Autodesk Fusion 360 part; units mm, degrees
sketch "Sketch1" plane through (0, 0, 0) normal (0, 1, 0) x (1, 0, 0)
  line L0 (-40.005, 0) -> (40.005, 0)
  line L1 (0, -29.21) -> (0, 0) construction
  line L2 (-1.524, -55.2004) -> (-1.524, -58.3802)
  line L3 (1.524, -55.2004) -> (1.524, -58.3802)
  line L4 (-1.524, -56.7903) -> (1.524, -56.7903) construction
  arc A0 (1.524, -55.2004) -> (-1.524, -55.2004) centre (0, -29.21) ccw
  arc A1 (40.005, 0) -> (29.1884, -28.0872) centre (67.2603, -26.6226) ccw
  arc A2 (-29.1884, -28.0872) -> (-40.005, 0) centre (-67.2603, -26.6226) ccw
  arc A3 (1.524, -58.3802) -> (29.1884, -28.0872) centre (0, -29.21) ccw
  arc A4 (-29.1884, -28.0872) -> (-1.524, -58.3802) centre (0, -29.21) ccw
  dimension "d1" = 52.07
  dimension "d2" = 29.21
  dimension "d3" = 80.01
  dimension "d4" = 58.42
  dimension "d5" = 3.048
  dimension "d7" = 38.1
extrude "Extrude1" add sketch "Sketch1" along normal blind 25.4
sketch "Sketch2" plane through (0, 0, 0) normal (0, 0, 1) x (1, 0, 0)
  circle A0 centre (0, 12.7) radius 3.302
  line L0 (-1.524, 25.4) -> (-29.21, 25.4)
  line L1 (-1.524, 0) -> (-29.21, 0)
  line L2 (-5.6643, 25.4) -> (-5.6643, 0) construction
  line L3 (-5.6643, 12.7) -> (0, 12.7) construction
  line L4 (1.524, 0) -> (1.524, 25.4) construction
  line L5 (-1.524, 0) -> (-1.524, 25.4) construction
  line L6 (0, 12.7) -> (0, 14.224) construction
  line L7 (0, 14.224) -> (-1.524, 14.224) construction
  line L8 (0, 14.224) -> (1.524, 14.224) construction
  dimension "d10" = 6.604
extrude "Extrude2" cut sketch "Sketch2" along normal blind 65.6387 and the other way blind -9.7561
Work out the finished part from the listing and answer in its coordinate system (mm). A direction names the side the tool comes from. Coordinates: 2 decimals unless noted, no trailing zeros. Write each loop counter-clockwise with the first axis right and the second up, starting at its lowest first coordinate (ties: lowest second). Pieces come first, ordered by that corner, then holes. Notation, with made-up numbers: (-22, 83) - (6, 83) arc R11 cw to (6, 91) - close; hole circle Ø9 at (-38, -35.5). An arc over 180 degrees is marked (long way). One line per question, with ' | ' between items.
1) For faces 1 (the face through (-1, 13, 0)), 2 (the face through (-3.3, 12.6, 56.7)), 3 (the face through (-1.524, 20, 57)), determine the directions among +Z, -Z, +X, -X, +Y, -Y from which every point of the face is accessible in a straight line to the end or side of a thin tool.
Checks:
face 1: -Z, +X, -X, +Y, -Y | face 2: +Z | face 3: +Z, +Y, -Y
2) Flat-ended cylindrical pins translate along their axes: P1, Ø1.6, axis at y = 7, z = 57, coming from the +X side; P2, Ø6, axis at x = -21, y = 20.5, coming from the +Z side; P3, Ø6, axis at x = -15.5, z = 13, coming from the +Y side; P4, Ø10, axis at x = 30, y = 10, coming from the +Z side. Find the tip coordinate at first contact, or state that the pin passes through.
Checks:
P1: x = 11.17 | P2: z = 52.21 | P3: through | P4: z = 44.32
3) Find section C-C, the plane x = 0. Determine the outline of the cut face in (y, z).
Checks:
outline: (0, 0) - (25.4, 0) - (25.4, 3.17) - (0, 3.17) - close
4) Consider probe 1 along X at (y, z) = (11.75, 28.5); probe 2 along X at (y, z) = (16.25, 7); probe 3 along Z at (x, y) = (-6.5, 6.5). Determine where each line is inside the solid, lowest interval first. Write a range as [from, to].
Checks:
probe 1: [-29.2, -26.03], [26.03, 29.2] | probe 2: [-34.6, -13.58], [13.58, 34.6] | probe 3: [0, 4], [54.42, 57.69]
5) Find section D-D, the plane y = 10.75. Determine the outline of the cut face in (x, z) (3 decimals), and give its area (3 significant figures).
Checks:
outline: (-40.005, 0) - (40.005, 0) arc R38.1 cw to (29.188, 28.087) arc R29.21 ccw to (2.665, 58.298) - (2.665, 55.108) arc R26.035 cw (long way) to (-2.665, 55.108) - (-2.665, 58.298) arc R29.21 ccw to (-29.188, 28.087) arc R38.1 cw to start | area: 1,080 mm2
6) Find section B-B, the plane x = -24. Determine the outline of the cut face in (y, z).
Checks:
outline: (0, 0) - (25.4, 0) - (25.4, 19.12) - (0, 19.12) - close; (0, 39.3) - (25.4, 39.3) - (25.4, 45.86) - (0, 45.86) - close
7) The mould has two halves that part along X. Classify faces 4 (the face through (-31.784, 12.522, 12.728)), 5 (the face through (1.524, 20, 57)), 6 (the face through (31.63, 12.52, 13.13)): +X half, -X half, draft (parallel to the pull), parting line (faces both ways), or undercut.
Checks:
face 4: -X half | face 5: undercut | face 6: +X half
8) Find section A-A, the plane z = 29.21. Determine the outline of the cut face in (x, y), and give its area (3 significant figures).
Checks:
outline: (-29.21, 0) - (-26.04, 0) - (-26.04, 25.4) - (-29.21, 25.4) - close; (26.04, 0) - (29.21, 0) - (29.21, 25.4) - (26.04, 25.4) - close | area: 161 mm2
